```python
from build123d import *

# Parameters (mm, degrees)
SKETCH_1_R               = 35
SKETCH_1_R_2             = 2.5
EXTRUDE_1_DEPTH          = 20
CUT_EXTRUDE_START        = -20
CUT_EXTRUDE_1_DEPTH      = 20
PATTERN_CIRCULAR_1_COUNT = 9
SKETCH_3_R               = 1.5
CUT_EXTRUDE_2_DEPTH      = 20


with BuildPart() as part:
    # 草图1 → 凸台-拉伸1 (new body)
    with BuildSketch(Plane.XY):
        Circle(SKETCH_1_R)
        Circle(SKETCH_1_R_2, mode=Mode.SUBTRACT)
    extrude(amount=EXTRUDE_1_DEPTH)

    # 草图2 → 切除-拉伸1 (cut)
    with BuildSketch(Plane.XY.offset(20).offset(CUT_EXTRUDE_START)):
        with BuildLine():
            Line((-1.5, 25), (1.5, 25))
            Line((1.5, 25), (1.5, 34.96784237))
            ThreePointArc((1.5, 34.96784237), (0, 35), (-1.5, 34.96784237))
            Line((-1.5, 34.96784237), (-1.5, 25))
        make_face()
    cut_extrude_1 = extrude(amount=CUT_EXTRUDE_1_DEPTH, mode=Mode.SUBTRACT)

    # 阵列(圆周)1: 切除-拉伸1 ×9 about axis
    pattern_circular_1_axis = Axis((0, 0, 0), (0, 0, 1))
    for i in range(1, PATTERN_CIRCULAR_1_COUNT):
        add(cut_extrude_1.rotate(pattern_circular_1_axis, i * 360 / PATTERN_CIRCULAR_1_COUNT), mode=Mode.SUBTRACT)

    # 草图3 → 切除-拉伸2 (cut)
    with BuildSketch(Plane.XY.offset(20)):
        with Locations((6.840402867, 18.793852416)):
            Circle(SKETCH_3_R)
        with Locations((-6.840402867, -18.793852416)):
            Circle(SKETCH_3_R)
    extrude(amount=-CUT_EXTRUDE_2_DEPTH, mode=Mode.SUBTRACT)


solid = part.part
```
Source: CAD feature listing. Evaluate the final solid. Frame: model axes, mm. A direction names the side the tool comes from. Give positions to 0.01 mm unless a question says otherwise; leave off trailing zeros. Order: outer loops, then holes, each group sorted by start corner. A loop starts at its lowest first (then second) coordinate and runs counter-clockwise, first axis right, second up. Notation, with made-up numbers: (20, 85) -> (74, 85) arc R16 ccw to (74, 111) -> close; hole circle Ø3 at (11.5, -3.75). An arc over 180 degrees is marked (long way). Use a Markdown table: item, result.
Q1. Section C-C (z = 4.5). State how many separate pieces and enclosed holes the cut face has, and give its area (3 significant figures).
A:
| item | result |
|---|---|
| separate pieces | 1 |
| enclosed holes | 3 |
| area | 3,540 mm^2 |
Q2. Pull-direction query (X, two-part tool) for faces 1 (the face through (7, 0, 20)), 2 (the face through (18.17, 23.99, 9.86)), 3 (the face through (29.337, 6.696, 9.86)); classes: +X half, -X half, draft (parallel to the pull), parting line (faces both ways), or undercut.
A:
| item | result |
|---|---|
| face 1 | draft |
| face 2 | undercut |
| face 3 | +X half |
Q3. Section A-A (y = 0). Return the cut outline in (x, z), and give its area (3 significant figures).
A:
| item | result |
|---|---|
| outline | (-35, 0) -> (-2.5, 0) -> (-2.5, 20) -> (-35, 20) -> close; (2.5, 0) -> (35, 0) -> (35, 20) -> (2.5, 20) -> close |
| area | 1,300 mm^2 |
Q4. First-contact query: P1, Ø11, axis at y = 29, z = 7, coming from the +X side; P2, Ø10, axis at y = -26, z = 3.5, coming from the -X side; P3, Ø0.9, axis at x = -0.5, z = 11.5, coming from the +Y side; P4, Ø4.5, axis at x = 0, y = 0, coming from the -Z side. Flat tips, straight axial feed; report the tip coordinate or a pass-through.
A:
| item | result |
|---|---|
| P1 | x = 25.94 |
| P2 | x = -28 |
| P3 | y = 25 |
| P4 | through |
Q5. Access query for faces 4 (the face through (26.78, -13.73, 9.86)), 5 (the face through (7, 0, 0)), 6 (the face through (-1.5, 30, 10)). Directions: +Z, -Z, +X, -X, +Y, -Y. A direction counts if a zero-diameter tool reaches every point of the face in a straight line with its end or side. Return the directions, or none.
A:
| item | result |
|---|---|
| face 4 | +Z, -Z |
| face 5 | -Z, +X, -X, +Y, -Y |
| face 6 | +Z, -Z, +Y |
Q6. Section B-B (x = 0). Return the cut outline in (y, z), and give its area (3 significant figures).
A:
| item | result |
|---|---|
| outline | (-35, 0) -> (-2.5, 0) -> (-2.5, 20) -> (-35, 20) -> close; (2.5, 0) -> (25, 0) -> (25, 20) -> (2.5, 20) -> close |
| area | 1,100 mm^2 |
Q7. Section D-D (y = 10.5). Return the cut outline in (x, z), and give its area (3 significant figures).
A:
| item | result |
|---|---|
| outline | (-33.39, 0) -> (33.39, 0) -> (33.39, 20) -> (-33.39, 20) -> close |
| area | 1,340 mm^2 |
Q8. Material intervals for line 1 (Y direction, x = -26, z = 7); line 2 (Y direction, x = -27.5, z = 6); line 3 (Y direction, x = 0, z = 8.5), sorted ascending. Write a range as [from, to].
A:
| item | result |
|---|---|
| line 1 | [-23.43, -16.74], [-13.28, 3.06], [6.11, 23.43] |
| line 2 | [-21.65, -17.61], [-14.15, 3.33], [6.37, 21.65] |
| line 3 | [-35, -2.5], [2.5, 25] |
